Work out the finished part from the listing and answer in its coordinate system (mm). Give positions to 0.01 mm unless a question says otherwise; leave off trailing zeros. Order: outer loops, then holes, each group sorted by start corner. A loop starts at its lowest first (then second) coordinate and runs counter-clockwise, first axis right, second up. Notation, with made-up numbers: (89, 14.25) -> (106, 14.25) arc R34 ccw to (106, 47.25) -> close; hole circle Ø10 at (39.25, 87). An arc over 180 degrees is marked (long way). Answer as CSV lines item,"result". Start each with the question number.
1. A cutting plane is placed at C-C (x = 544.5). Give the vertices of the cut face in (y, z).
2. A cutting plane is placed at B-B (z = 0.95). State how many separate pieces and enclosed holes the cut face has, then the cut area to 3 significant figures.
3. A flat-ended cylindrical pin translates along its axis: pin 1 (3 mm diameter, centred on x = 12.7, y = -88.9, fed in from +Z). Find the tip coordinate at first contact, or state that the pin passes through.
4. A cutting plane is placed at A-A (y = -240). Give the vertices of the cut face in (x, z), then the cut area to 3 significant figures.
5. Find the intervals of material crossed by L1, parallel to X at y = -283, z = 2.8; L2, parallel to X at y = -26, z = 0.3 (3 decimals); L3, parallel to Y at x = 368.5, z = 4.3, in increasing order.
from build123d import *

# Parameters (mm, degrees)
SKETCH1_W           = 752.475
SKETCH1_H           = 381
BOSS_EXTRUDE1_DEPTH = 4.7625
SKETCH2_W           = 8.379539034
SKETCH2_H           = 75.702321135
CUT_EXTRUDE1_DEPTH  = 10.668
SKETCH3_W           = 9.682653374
SKETCH3_H           = 75.707969864
CUT_EXTRUDE2_DEPTH  = 10.668
SKETCH4_W           = 166.904258103
SKETCH4_H           = 154.899111528
CUT_EXTRUDE3_DEPTH  = 10.668
SKETCH5_W           = 167.650404688
SKETCH5_H           = 154.899111528
CUT_EXTRUDE5_DEPTH  = 10.668
SKETCH6_R           = 2.667
CUT_EXTRUDE6_DEPTH  = 844.446682981


with BuildPart() as part:
    # Sketch1 → Boss-Extrude1 (new body)
    with BuildSketch(Plane.XY):
        with Locations((376.2375, -190.5)):
            Rectangle(SKETCH1_W, SKETCH1_H)
    extrude(amount=BOSS_EXTRUDE1_DEPTH)

    # Sketch2 → Cut-Extrude1 (cut)
    with BuildSketch(Plane(origin=(0, 0, 0), x_dir=(-1, 0, 0), z_dir=(0, 0, -1))):
        with Locations((-748.285230483, -263.95204904)):
            Rectangle(SKETCH2_W, SKETCH2_H)
    extrude(amount=-CUT_EXTRUDE1_DEPTH, mode=Mode.SUBTRACT)

    # Sketch3 → Cut-Extrude2 (cut)
    with BuildSketch(Plane(origin=(0, 0, 0), x_dir=(-1, 0, 0), z_dir=(0, 0, -1))):
        with Locations((-4.841326687, -263.949224675)):
            Rectangle(SKETCH3_W, SKETCH3_H)
    extrude(amount=-CUT_EXTRUDE2_DEPTH, mode=Mode.SUBTRACT)

    # Sketch4 → Cut-Extrude3 (cut)
    with BuildSketch(Plane(origin=(0, 0, 0), x_dir=(-1, 0, 0), z_dir=(0, 0, -1))):
        with Locations((-589.168581759, -303.550444236)):
            Rectangle(SKETCH4_W, SKETCH4_H)
    extrude(amount=-CUT_EXTRUDE3_DEPTH, mode=Mode.SUBTRACT)

    # Sketch5 → Cut-Extrude5 (cut)
    with BuildSketch(Plane(origin=(0, 0, 0), x_dir=(-1, 0, 0), z_dir=(0, 0, -1))):
        with Locations((-166.139683848, -303.550444236)):
            Rectangle(SKETCH5_W, SKETCH5_H)
    extrude(amount=-CUT_EXTRUDE5_DEPTH, mode=Mode.SUBTRACT)

    # Sketch6 → Cut-Extrude6 (cut, through all)
    with BuildSketch(Plane.XY.offset(4.7625)):
        with Locations((12.7, -12.7)):
            Circle(SKETCH6_R)
        with Locations((12.7, -25.4)):
            Circle(SKETCH6_R)
        with Locations((12.7, -38.1)):
            Circle(SKETCH6_R)
        with Locations((12.7, -50.8)):
            Circle(SKETCH6_R)
        with Locations((12.7, -63.5)):
            Circle(SKETCH6_R)
        with Locations((12.7, -76.2)):
            Circle(SKETCH6_R)
        with Locations((12.7, -88.9)):
            Circle(SKETCH6_R)
        with Locations((12.7, -101.6)):
            Circle(SKETCH6_R)
        with Locations((12.7, -114.3)):
            Circle(SKETCH6_R)
        with Locations((12.7, -127)):
            Circle(SKETCH6_R)
        with Locations((12.7, -139.7)):
            Circle(SKETCH6_R)
        with Locations((12.7, -152.4)):
            Circle(SKETCH6_R)
        with Locations((12.7, -165.1)):
            Circle(SKETCH6_R)
        with Locations((12.7, -177.8)):
            Circle(SKETCH6_R)
        with Locations((12.7, -190.5)):
            Circle(SKETCH6_R)
        with Locations((12.7, -203.2)):
            Circle(SKETCH6_R)
        with Locations((12.7, -215.9)):
            Circle(SKETCH6_R)
        with Locations((12.7, -304.8)):
            Circle(SKETCH6_R)
        with Locations((12.7, -317.5)):
            Circle(SKETCH6_R)
        with Locations((12.7, -330.2)):
            Circle(SKETCH6_R)
        with Locations((12.7, -342.9)):
            Circle(SKETCH6_R)
        with Locations((12.7, -355.6)):
            Circle(SKETCH6_R)
        with Locations((12.7, -368.3)):
            Circle(SKETCH6_R)
        with Locations((739.775, -368.3)):
            Circle(SKETCH6_R)
        with Locations((739.775, -355.6)):
            Circle(SKETCH6_R)
        with Locations((739.775, -342.9)):
            Circle(SKETCH6_R)
        with Locations((739.775, -330.2)):
            Circle(SKETCH6_R)
        with Locations((739.775, -304.8)):
            Circle(SKETCH6_R)
        with Locations((739.775, -317.5)):
            Circle(SKETCH6_R)
        with Locations((739.775, -215.9)):
            Circle(SKETCH6_R)
        with Locations((739.775, -203.2)):
            Circle(SKETCH6_R)
        with Locations((739.775, -190.5)):
            Circle(SKETCH6_R)
        with Locations((739.775, -177.8)):
            Circle(SKETCH6_R)
        with Locations((739.775, -165.1)):
            Circle(SKETCH6_R)
        with Locations((739.775, -152.4)):
            Circle(SKETCH6_R)
        with Locations((739.775, -139.7)):
            Circle(SKETCH6_R)
        with Locations((739.775, -127)):
            Circle(SKETCH6_R)
        with Locations((739.775, -114.3)):
            Circle(SKETCH6_R)
        with Locations((739.775, -101.6)):
            Circle(SKETCH6_R)
        with Locations((739.775, -88.9)):
            Circle(SKETCH6_R)
        with Locations((739.775, -76.2)):
            Circle(SKETCH6_R)
        with Locations((739.775, -63.5)):
            Circle(SKETCH6_R)
        with Locations((739.775, -50.8)):
            Circle(SKETCH6_R)
        with Locations((739.775, -38.1)):
            Circle(SKETCH6_R)
        with Locations((739.775, -25.4)):
            Circle(SKETCH6_R)
        with Locations((739.775, -12.7)):
            Circle(SKETCH6_R)
        with Locations((25.4, -368.3)):
            Circle(SKETCH6_R)
        with Locations((38.1, -368.3)):
            Circle(SKETCH6_R)
        with Locations((50.8, -368.3)):
            Circle(SKETCH6_R)
        with Locations((63.5, -368.3)):
            Circle(SKETCH6_R)
        with Locations((76.2, -368.3)):
            Circle(SKETCH6_R)
        with Locations((88.9, -368.3)):
            Circle(SKETCH6_R)
        with Locations((101.6, -368.3)):
            Circle(SKETCH6_R)
        with Locations((114.3, -368.3)):
            Circle(SKETCH6_R)
        with Locations((127, -368.3)):
            Circle(SKETCH6_R)
        with Locations((139.7, -368.3)):
            Circle(SKETCH6_R)
        with Locations((152.4, -368.3)):
            Circle(SKETCH6_R)
        with Locations((165.1, -368.3)):
            Circle(SKETCH6_R)
        with Locations((177.8, -368.3)):
            Circle(SKETCH6_R)
        with Locations((190.5, -368.3)):
            Circle(SKETCH6_R)
        with Locations((203.2, -368.3)):
            Circle(SKETCH6_R)
        with Locations((215.9, -368.3)):
            Circle(SKETCH6_R)
        with Locations((228.6, -368.3)):
            Circle(SKETCH6_R)
        with Locations((241.3, -368.3)):
            Circle(SKETCH6_R)
        with Locations((266.7, -368.3)):
            Circle(SKETCH6_R)
        with Locations((279.4, -368.3)):
            Circle(SKETCH6_R)
        with Locations((292.1, -368.3)):
            Circle(SKETCH6_R)
        with Locations((304.8, -368.3)):
            Circle(SKETCH6_R)
        with Locations((317.5, -368.3)):
            Circle(SKETCH6_R)
        with Locations((330.2, -368.3)):
            Circle(SKETCH6_R)
        with Locations((342.9, -368.3)):
            Circle(SKETCH6_R)
        with Locations((355.6, -368.3)):
            Circle(SKETCH6_R)
        with Locations((368.3, -368.3)):
            Circle(SKETCH6_R)
        with Locations((381, -368.3)):
            Circle(SKETCH6_R)
        with Locations((393.7, -368.3)):
            Circle(SKETCH6_R)
        with Locations((406.4, -368.3)):
            Circle(SKETCH6_R)
        with Locations((419.1, -368.3)):
            Circle(SKETCH6_R)
        with Locations((431.8, -368.3)):
            Circle(SKETCH6_R)
        with Locations((444.5, -368.3)):
            Circle(SKETCH6_R)
        with Locations((457.2, -368.3)):
            Circle(SKETCH6_R)
        with Locations((469.9, -368.3)):
            Circle(SKETCH6_R)
        with Locations((482.6, -368.3)):
            Circle(SKETCH6_R)
        with Locations((495.3, -368.3)):
            Circle(SKETCH6_R)
        with Locations((520.7, -368.3)):
            Circle(SKETCH6_R)
        with Locations((533.4, -368.3)):
            Circle(SKETCH6_R)
        with Locations((546.1, -368.3)):
            Circle(SKETCH6_R)
        with Locations((558.8, -368.3)):
            Circle(SKETCH6_R)
        with Locations((571.5, -368.3)):
            Circle(SKETCH6_R)
        with Locations((584.2, -368.3)):
            Circle(SKETCH6_R)
        with Locations((596.9, -368.3)):
            Circle(SKETCH6_R)
        with Locations((609.6, -368.3)):
            Circle(SKETCH6_R)
        with Locations((622.3, -368.3)):
            Circle(SKETCH6_R)
        with Locations((635, -368.3)):
            Circle(SKETCH6_R)
        with Locations((647.7, -368.3)):
            Circle(SKETCH6_R)
        with Locations((660.4, -368.3)):
            Circle(SKETCH6_R)
        with Locations((685.8, -368.3)):
            Circle(SKETCH6_R)
        with Locations((698.5, -368.3)):
            Circle(SKETCH6_R)
        with Locations((711.2, -368.3)):
            Circle(SKETCH6_R)
        with Locations((723.9, -368.3)):
            Circle(SKETCH6_R)
    extrude(amount=-CUT_EXTRUDE6_DEPTH, mode=Mode.SUBTRACT)


solid = part.part
Answer sheet:
1,outline,"(-226.1, 0) -> (0, 0) -> (0, 4.76) -> (-226.1, 4.76) -> close"
2,separate pieces,"1"
2,enclosed holes,"74"
2,area,"232,000 mm^2"
3,pin 1,"passes through"
4,outline,"(9.68, 0) -> (82.31, 0) -> (82.31, 4.76) -> (9.68, 4.76) -> close; (249.96, 0) -> (505.72, 0) -> (505.72, 4.76) -> (249.96, 4.76) -> close; (672.62, 0) -> (744.1, 0) -> (744.1, 4.76) -> (672.62, 4.76) -> close"
4,area,"1,900 mm^2"
5,L1,"x = 9.68 to 82.31, 249.96 to 505.72, 672.62 to 744.1"
5,L2,"x = 0 to 10.101, 15.299 to 737.176, 742.374 to 752.475"
5,L3,"y = -381 to -370.96, -365.64 to 0"
